from build123d import *

# Parameters (mm, degrees)
F0_W     = 50
F0_H     = 45
F0_R     = 1.6
F1_DEPTH = 3
F3_D     = 2.5


with BuildPart() as f1:
    # F0 (on Top) → F1 (new body)
    with BuildSketch(Plane.XY):
        Rectangle(F0_W, F0_H)
        with Locations((-22, -19.5)):
            Circle(F0_R, mode=Mode.SUBTRACT)
        with Locations((22, -19.5)):
            Circle(F0_R, mode=Mode.SUBTRACT)
        with Locations((-22, 19.5)):
            Circle(F0_R, mode=Mode.SUBTRACT)
        with Locations((22, 19.5)):
            Circle(F0_R, mode=Mode.SUBTRACT)
    extrude(amount=F1_DEPTH)

    # F3 (through all)
    with Locations(Plane.XY.offset(3)):
        with Locations((-15, 12.5), (15, 12.5), (15, -12.5), (-15, -12.5)):
            Hole(F3_D / 2)


solid = f1.part
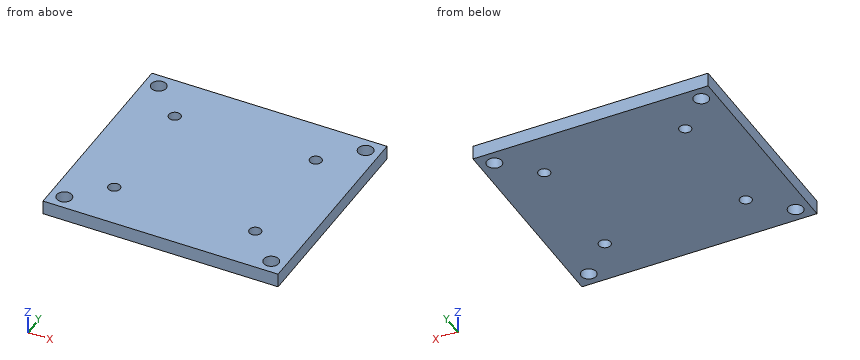
Here's how the part is built. I have some questions about the finished solid (model axes, mm). Give positions to 0.01 mm unless a question says otherwise; leave off trailing zeros. Order: outer loops, then holes, each group sorted by start corner. A loop starts at its lowest first (then second) coordinate and runs counter-clockwise, first axis right, second up. Notation, with made-up numbers: M -12.5,-28 L 31.5,-28 A19 cw 31.5,4 Z; hole C -11.75,72 d11. An arc over 180 degrees is marked long. Answer as a JSON object with one key per item and string values. Group by question number.
1) Suppose I cut it at B-B, the plane x = -15. Write out the boundary of the cut face in (y, z).
2) Suppose I cut it at A-A, the plane y = 19.5. Write out the boundary of the cut face in (x, z), plus the area to 3 significant figures.
3) Please list where these lines run through material, in increasing order: L1, parallel to Y at x = 22, z = 1.2; L2, parallel to Y at x = -15, z = 0.75; L3, parallel to X at y = 13, z = 1.8. Write a range as [from, to].
4) I'm going to push a flat-ended pin straight in: pin 1 Ø1.9 at (x, y) = (22, 19.5) entering from +Z. Where does the tip first touch, or does it pass through?
5) Suppose I cut it at C-C, the plane z = 1.9. Count the separate pieces of the cut face and the enclosed holes in it, plus the area to 3 significant figures.
Results found:
{
 "1": {"outline": "M -22.5,0 L -13.75,0 L -13.75,3 L -22.5,3 Z; M -11.25,0 L 11.25,0 L 11.25,3 L -11.25,3 Z; M 13.75,0 L 22.5,0 L 22.5,3 L 13.75,3 Z"},
 "2": {"outline": "M -25,0 L -23.6,0 L -23.6,3 L -25,3 Z; M -20.4,0 L 20.4,0 L 20.4,3 L -20.4,3 Z; M 23.6,0 L 25,0 L 25,3 L 23.6,3 Z", "area": "131 mm²"},
 "3": {"L1": "[-22.5, -21.1], [-17.9, 17.9], [21.1, 22.5]", "L2": "[-22.5, -13.75], [-11.25, 11.25], [13.75, 22.5]", "L3": "[-25, -16.15], [-13.85, 13.85], [16.15, 25]"},
 "4": {"pin 1": "through"},
 "5": {"separate pieces": "1", "enclosed holes": "8", "area": "2,200 mm²"}
}
